Verification items for the finished model (mm, model axes). Face numbers are marked on the shaded views. Coordinates: 2 decimals unless noted, no trailing zeros. One line per item, written item: value. Start each with the question number.
(1) Gauge pin test, flat ends, axial feed: P1, Ø2, axis at y = -9.5, z = -5, coming from the -X side; P2, Ø5, axis at x = -0.5, y = -6, coming from the -Z side; P3, Ø4, axis at y = -4.5, z = -5.5, coming from the -X side. Record the tip position at first contact, or that the pin passes through.
(2) Thickness scan on probe 1 along Y at (x, z) = (2.25, 1); probe 2 along X at (y, z) = (2.5, 0.25); probe 3 along X at (y, z) = (4, -2). Record the ranges inside material, lowest first. Write a range as [from, to].
(3) Section check A-A (z = 0). Count the separate pieces of the cut face and the enclosed holes in it, plus the area to 3 significant figures.
(4) Draft check along Z on the marked faces 1, 2, 3 and 4. Enter one of: +Z half, -Z half, draft (parallel to the pull), parting line (faces both ways), or undercut.
Autodesk Inventor part; units mm, degrees
ref_plane "YZ Plane" through (0, 0, 0) normal (1, 0, 0) x (0, 1, 0)
ref_plane "XZ Plane" through (0, 0, 0) normal (0, 1, 0) x (-1, 0, 0)
ref_plane "XY Plane" through (0, 0, 0) normal (0, 0, 1) x (1, 0, 0)
sketch "Sketch1" plane through (0, 0, 0) normal (0, 0, 1) x (1, 0, 0)
  line L0 (-1.2723, 5.8241) -> (-1.2723, -4.8856)
  line L1 (1.2277, 5.0871) -> (1.2277, 3.0871)
  line L2 (5.7277, 5.0871) -> (5.7277, -0.9129)
  line L3 (3.9777, -0.9129) -> (3.9777, -11.9129)
  line L4 (1.2277, 5.0871) -> (5.7277, 5.0871)
  line L5 (5.7277, -0.9129) -> (3.9777, -0.9129)
  line L6 (0.7277, 3.0871) -> (0.7277, -7.8065)
  line L7 (1.2277, 3.0871) -> (0.7277, 3.0871)
  line L8 (0.7277, -7.8065) -> (2.9777, -7.8065)
  line L9 (2.9777, -7.8065) -> (2.9777, -10.8065)
  line L10 (0.0277, -11.0469) -> (-0.4723, -11.9129)
  line L11 (-0.4723, -11.9129) -> (3.9777, -11.9129)
  line L12 (2.9777, -10.8065) -> (0.1665, -10.8065)
  line L13 (0.1665, -10.8065) -> (0.0277, -11.0469)
  point P0 (0, 0)
  dimension "d0" = 5
  dimension "d1" = 6
  dimension "d2" = 14
  dimension "d3" = 11
  dimension "d4" = 2
  dimension "d5" = 4
  dimension "d6" = 10.5
  dimension "d7" = 3
  dimension "d8" = 8.5
  dimension "d11" = 0.8
revolve "Revolution1" add sketch "Sketch1" angle 360 about axis through (-1.2723, 5.8241, 0) along (0, -1, 0)
fillet "Fillet1" radius 0.5 1 edges at (-8.2723, -0.9129, 0)
sketch "Sketch4" plane through (-1.2723, 5.0871, 0) normal (0, 1, 0) x (1, 0, 0)
  circle A0 centre (-4.85, 0) radius 0.65
  circle A1 centre (4.85, 0) radius 0.65
  circle A2 centre (0, 0) radius 7
  point P0 (1.2723, 0)
  dimension "d25" = 1.3
  dimension "d26" = 1.3
  dimension "d28" = 1.5
  dimension "d29" = 1.5
  dimension "d30" = 11
sketch "Sketch5" plane through (0, 0, 0) normal (0, 0, 1) x (1, 0, 0)
  line L0 (-8.2723, 5.0871) -> (5.7277, 5.0871)
  line L1 (3.5777, 5.0871) -> (1.9777, -8.3912)
  line L2 (-8.2723, 5.0871) -> (-8.2723, -0.4129)
  line L3 (5.7277, 5.0871) -> (5.7277, -0.4129)
  line L4 (-6.1223, 5.0871) -> (-4.5223, -8.3912)
  line L5 (-5.5223, -10.8065) -> (-5.5223, -7.8065)
  line L6 (2.9777, -10.8065) -> (2.9777, -7.8065)
  point P0 (0, 0)
  dimension "d31" = 2.15
  dimension "d32" = 2.15
  dimension "d33" = 1
  dimension "d34" = 1
sweep "Sweep2" cut profiles "Sketch4" path "Sketch5" path curves L1 contours A1
sketch "Sketch6" plane through (-1.2723, 5.0871, 0) normal (0, 1, 0) x (1, 0, 0)
  circle A0 centre (-4.85, 0) radius 0.65
  circle A1 centre (0, 0) radius 7
  circle A2 centre (4.85, 0) radius 0.65
  point P0 (1.2723, 0)
  dimension "d37" = 1.3
  dimension "d38" = 11
sketch "Sketch7" plane through (0, 0, 0) normal (0, 0, 1) x (1, 0, 0)
  line L0 (-8.2723, 5.0871) -> (5.7277, 5.0871)
  line L1 (-6.1223, 5.0871) -> (-4.5223, -8.1262)
  line L2 (-5.5223, -10.8065) -> (2.9777, -10.8065)
  line L3 (-5.5223, -7.8065) -> (2.9777, -7.8065)
  line L4 (-5.5223, -10.8065) -> (-5.5223, -7.8065)
  line L5 (-8.2723, 5.0871) -> (-8.2723, -0.4129)
  point P0 (0, 0)
  dimension "d39" = 1
  dimension "d40" = 2.15
sweep "Sweep3" cut profiles "Sketch6" path "Sketch7" path curves L1 contours A0
properties part number "Musab4" material "Steel, Alloy"
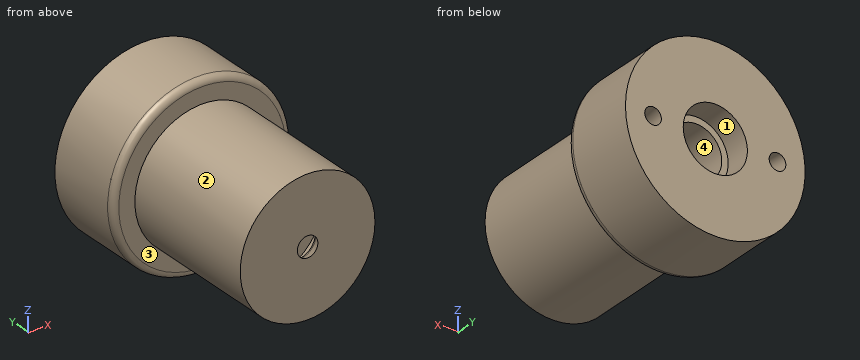
Responses:
1. P1: stops at x = -4.67
1. P2: stops at z = -5.25
1. P3: stops at x = -5.19
2. probe 1: y = [-11.91, -10.81], [-7.81, 5.09]
2. probe 2: x = [-8.27, -6.41], [-5.21, -3.26], [0.71, 2.67], [3.87, 5.72]
2. probe 3: x = [-7.98, -2.77], [0.23, 5.44]
3. separate pieces: 4
3. enclosed holes: 0
3. area: 84.3 mm²
4. face 1: undercut
4. face 2: parting line
4. face 3: draft
4. face 4: undercut
